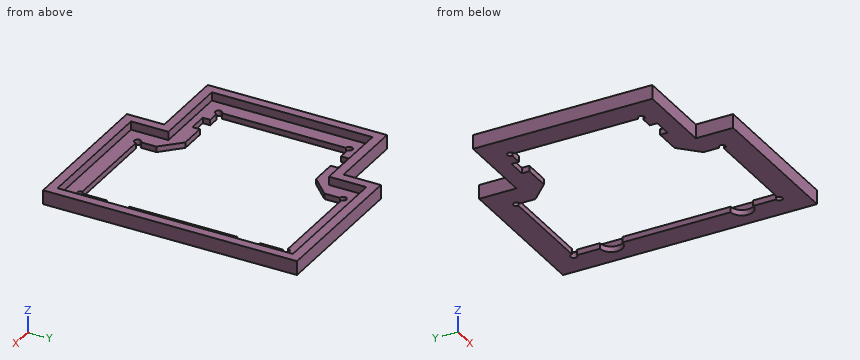
```python
from build123d import *

# Parameters (mm, degrees)
F1_DEPTH  = 3
F3_DEPTH  = 3
F5_DEPTH  = 3.001
F6_R      = 1.75
F6_R_2    = 6
F6_W      = 10
F6_H      = 4
F7_DEPTH  = 25
F9_DEPTH  = 4.5
F11_DEPTH = 7.501


with BuildPart() as f1:
    # F0 (on Top) → F1 (new body)
    with BuildSketch(Plane.XY):
        Polygon((56.5, 63), (-14.5, 63), (-14.5, 43), (-56.5, 43), (-56.5, -43), (-14.5, -43), (-14.5, -63), (56.5, -63), align=None)
    extrude(amount=F1_DEPTH)

    # F2 (on face) → F3 (join, through all)
    with BuildSketch(Plane.XY.offset(3)):
        Polygon((-19.5, -68), (61.5, -68), (61.5, 68), (-19.5, 68), (-19.5, 48), (-61.5, 48), (-61.5, -48), (-19.5, -48), align=None)
        Polygon((-14.5, 63), (56.5, 63), (56.5, -63), (-14.5, -63), (-14.5, -43), (-56.5, -43), (-56.5, 43), (-14.5, 43), align=None, mode=Mode.SUBTRACT)
    extrude(amount=-F3_DEPTH)

    # F4 (on face) → F5 (cut, through all)
    with BuildSketch(Plane.XY.offset(3)):
        Polygon((-6.5, 55), (-6.5, 35), (-48.5, 35), (-48.5, -35), (-6.5, -35), (-6.5, -55), (48.5, -55), (48.5, 55), align=None)
    extrude(amount=-F5_DEPTH, mode=Mode.SUBTRACT)

    # F6 (on face) → F7 (cut)
    with BuildSketch(Plane.XY.offset(3)):
        with Locations((-48.5, 35)):
            Circle(F6_R)
        with Locations((-6.5, 55)):
            Circle(F6_R)
        with Locations((48.5, 55)):
            Circle(F6_R)
        with Locations((48.5, -55)):
            Circle(F6_R)
        with Locations((-6.5, -55)):
            Circle(F6_R)
        with Locations((-48.5, -35)):
            Circle(F6_R)
        with Locations((48.5, 35)):
            Circle(F6_R_2)
        with Locations((48.5, -35)):
            Circle(F6_R_2)
        with Locations((-35.5, 37)):
            Rectangle(F6_W, F6_H)
        with Locations((-35.5, -37)):
            Rectangle(F6_W, F6_H)
    extrude(amount=-F7_DEPTH, mode=Mode.SUBTRACT)

    # F8 (on face) → F9 (join)
    with BuildSketch(Plane.XY.offset(3)):
        Polygon((-19.5, -48), (-19.5, -68), (61.5, -68), (61.5, 68), (-19.5, 68), (-19.5, 48), (-61.5, 48), (-61.5, -48), align=None)
        Polygon((-14.5, 43), (-14.5, 63), (56.5, 63), (56.5, -63), (-14.5, -63), (-14.5, -43), (-56.5, -43), (-56.5, 43), align=None, mode=Mode.SUBTRACT)
    extrude(amount=F9_DEPTH)

    # F10 (on face) → F11 (cut, through all)
    with BuildSketch(Plane(origin=(0, 0, 0), x_dir=(1, 0, 0), z_dir=(0, 0, -1))):
        Polygon((-6.5, 35), (-6.5, 45), (-16.5, 35), align=None)
        Polygon((-16.5, -35), (-6.5, -45), (-6.5, -35), align=None)
    extrude(amount=-F11_DEPTH, mode=Mode.SUBTRACT)


solid = f1.part
```
CAD build for the part. Positions are in the model's coordinates, mm. Round coordinates to 2 decimals unless told otherwise and drop trailing zeros. Loops run counter-clockwise (first coordinate to the right, second up) from the corner with the lowest first, then second, coordinate; pieces in that order, holes last. Notation, with made-up numbers: (61, 34.5) - (72, 34.5) arc R33 cw to (72, 63.5) - close; hole circle Ø1 at (48, 80.5). An arc over 180 degrees is marked (long way). Return JSON: item names as keys, results as strings. Group by question number.
Q1. Band-saw the part on B-B on y = 11.5. Give the cut face in (x, z), plus the area to 3 significant figures.
Q2. Band-saw the part on C-C on z = 6. Give the cut face in (x, y), plus the area to 3 significant figures.
Q3. Drill centre lines: line 1 along X through (y, z) = (19.5, 7.25); line 2 along Y through (x, z) = (8.5, 5.5); line 3 along Y through (x, z) = (-23, 1.5). Where is each one in solid material? Low to high. Write a range as [from, to].
Q4. Band-saw the part on A-A on x = -44.5. Give the cut face in (y, z), plus the area to 3 significant figures.
Q5. Flat gauge pins, fed straight in: pin 1 Ø3 at (x, y) = (48.5, -48.5) entering from +Z; pin 2 Ø4.5 at (x, y) = (48.5, -55) entering from -Z; pin 3 Ø2 at (x, z) = (-40, 6.5) entering from -Y; pin 4 Ø2.5 at (y, z) = (49.5, 2) entering from -X. Where does each tip first touch, or does it go through?
Solutions:
{
 "1": {"outline": "(-61.5, 0) - (-48.5, 0) - (-48.5, 3) - (-56.5, 3) - (-56.5, 7.5) - (-61.5, 7.5) - close; (48.5, 0) - (61.5, 0) - (61.5, 7.5) - (56.5, 7.5) - (56.5, 3) - (48.5, 3) - close", "area": "123 mm^2"},
 "2": {"outline": "(-61.5, -48) - (-19.5, -48) - (-19.5, -68) - (61.5, -68) - (61.5, 68) - (-19.5, 68) - (-19.5, 48) - (-61.5, 48) - close; hole (-56.5, -43) - (-14.5, -43) - (-14.5, -63) - (56.5, -63) - (56.5, 63) - (-14.5, 63) - (-14.5, 43) - (-56.5, 43) - close", "area": "2,490 mm^2"},
 "3": {"line 1": "x = [-61.5, -56.5], [56.5, 61.5]", "line 2": "y = [-68, -63], [63, 68]", "line 3": "y = [-48, -35], [35, 48]"},
 "4": {"outline": "(-48, 0) - (-35, 0) - (-35, 3) - (-43, 3) - (-43, 7.5) - (-48, 7.5) - close; (35, 0) - (48, 0) - (48, 7.5) - (43, 7.5) - (43, 3) - (35, 3) - close", "area": "123 mm^2"},
 "5": {"pin 1": "stops at z = 3", "pin 2": "stops at z = 0", "pin 3": "stops at y = -48", "pin 4": "stops at x = -19.5"}
}
